Could you check a few things on this drawing? It's one solid part, dimensions in mm from its lowest x, y, z. A direction names the side the tool comes from. Round coordinates to 2 decimals unless told otherwise and drop trailing zeros. Write each loop counter-clockwise with the first axis right and the second up, starting at its lowest first coordinate (ties: lowest second). Pieces come first, ordered by that corner, then holes. Notation, with made-up numbers: (35, -31.5) -> (72, -31.5) arc R26 ccw to (72, 0.5) -> close; hole circle Ø8 at (-3, -19.5). An arc over 180 degrees is marked (long way). Put each result on its own line as item: value. Start each with the question number.
1) We'd pull the mould along Z, two halves only. Please class the marked faces 3, 4 and 5: released by +Z, released by -Z, zero draft, split by the parting line, or undercut.
2) I want a section at D-D, the plane z = 31. List the corners of the cut face in (x, y) for me, then the cut area to 3 significant figures.
3) I want a section at B-B, the plane x = 53. List the corners of the cut face in (y, z) for me, then the cut area to 3 significant figures.
4) Which directions (+Z, -Z, +X, -X, +Y, -Y) give clear straight access to the entire face, cutting with the end or side of a thin tool? Please do the marked faces 1 and 2.
5) Will these pins go through, and if not, where does the flat tip stop? P1, Ø5, axis at y = 57, z = 42, coming from the -X side; P2, Ø4, axis at x = 33.5, z = 22, coming from the +Y side.
6) I want a section at A-A, the plane y = 15.5. List the corners of the cut face in (x, z) for me, then the cut area to 3 significant figures.
7) I want a section at C-C, the plane z = 56. List the corners of the cut face in (x, y) for me.
8) If I drill on line 1 along Y through (x, z) = (0.9, 56); line 2 along Y through (x, z) = (0.4, 9); line 3 along X through (y, z) = (63.5, 50), over which ranges is the centre line in solid material (lowest first)? Write a range as [from, to].
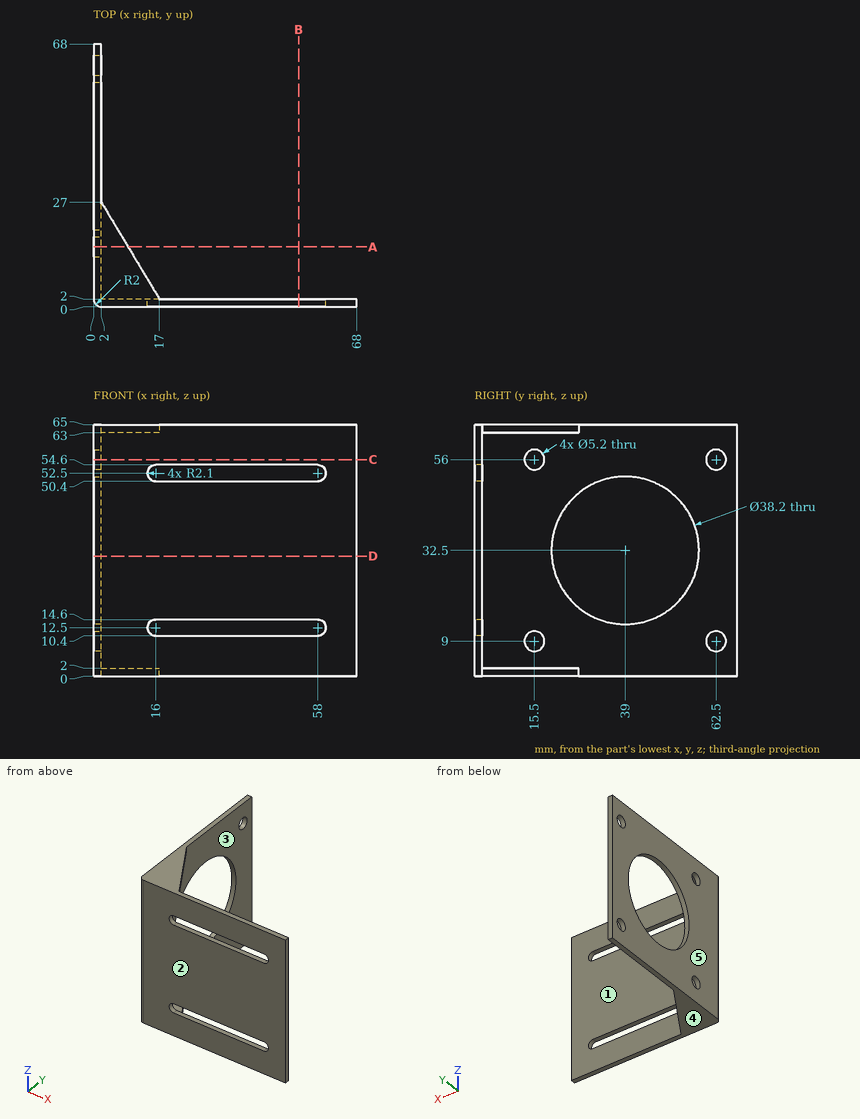
Findings:
1. face 3: undercut
1. face 4: released by -Z
1. face 5: zero draft
2. outline: (0, 2) arc R2 ccw to (2, 0) -> (68, 0) -> (68, 2) -> (2, 2) -> (2, 19.96) -> (0, 19.96) -> close; (0, 58.04) -> (2, 58.04) -> (2, 68) -> (0, 68) -> close
2. area: 191 mm2
3. outline: (0, 0) -> (2, 0) -> (2, 10.4) -> (0, 10.4) -> close; (0, 14.6) -> (2, 14.6) -> (2, 50.4) -> (0, 50.4) -> close; (0, 54.6) -> (2, 54.6) -> (2, 65) -> (0, 65) -> close
3. area: 113 mm2
4. face 1: +X, +Y
4. face 2: +Z, -Z, +X, -X, -Y
5. P1: stops at x = 0
5. P2: stops at y = 2
6. outline: (0, 0) -> (8.9, 0) -> (8.9, 2) -> (2, 2) -> (2, 6.4) -> (0, 6.4) -> close; (0, 11.6) -> (2, 11.6) -> (2, 53.4) -> (0, 53.4) -> close; (0, 58.6) -> (2, 58.6) -> (2, 63) -> (8.9, 63) -> (8.9, 65) -> (0, 65) -> close
6. area: 137 mm2
7. outline: (0, 2) arc R2 ccw to (2, 0) -> (68, 0) -> (68, 2) -> (2, 2) -> (2, 12.9) -> (0, 12.9) -> close; (0, 18.1) -> (2, 18.1) -> (2, 59.9) -> (0, 59.9) -> close; (0, 65.1) -> (2, 65.1) -> (2, 68) -> (0, 68) -> close
8. line 1: y = [0.33, 12.9], [18.1, 59.9], [65.1, 68]
8. line 2: y = [0.8, 12.9], [18.1, 59.9], [65.1, 68]
8. line 3: x = [0, 2]
